```python
from build123d import *

# Parameters (mm, degrees)
SKETCH1_R           = 32.5
BOSS_EXTRUDE1_DEPTH = 2.25
SKETCH15_W          = 12.75
SKETCH15_H          = 3.5
CUT_EXTRUDE6_DEPTH  = 17
SKETCH17_W          = 21.5
SKETCH17_H          = 3.5
CUT_EXTRUDE7_DEPTH  = 12
SKETCH19_R          = 1
CUT_EXTRUDE9_DEPTH  = 16
FILLET4_R           = 0.5
FILLET5_R           = 0.5
SKETCH21_R          = 6.125
CUT_EXTRUDE11_DEPTH = 13
FILLET8_R           = 0.75


with BuildPart() as part:
    # Sketch1 → Boss-Extrude1 (new body)
    with BuildSketch(Plane(origin=(0, 0, 0), x_dir=(1, 0, 0), z_dir=(0, 1, 0))):
        Circle(SKETCH1_R)
    extrude(amount=BOSS_EXTRUDE1_DEPTH)

    # Sketch15 → Cut-Extrude6 (cut)
    with BuildSketch(Plane(origin=(0.067128405, 2.25, -0.501790944), x_dir=(1, 0, 0), z_dir=(0, 1, 0))):
        Polygon((-13.916501725, 15.395911949), (-20.291501725, 4.354088051), (-23.322590638, 6.104088051), (-16.947590638, 17.145911949), align=None)
        with Locations((0, 21.5)):
            Rectangle(SKETCH15_W, SKETCH15_H)
        Polygon((-20.291501725, -4.354088051), (-13.916501725, -15.395911949), (-16.947590638, -17.145911949), (-23.322590638, -6.104088051), align=None)
        with Locations((0, -21.5)):
            Rectangle(SKETCH15_W, SKETCH15_H)
        Polygon((13.916501725, -15.395911949), (20.291501725, -4.354088051), (23.322590638, -6.104088051), (16.947590638, -17.145911949), align=None)
        Polygon((20.291501725, 4.354088051), (13.916501725, 15.395911949), (16.947590638, 17.145911949), (23.322590638, 6.104088051), align=None)
    extrude(amount=-CUT_EXTRUDE6_DEPTH, mode=Mode.SUBTRACT)

    # Sketch17 → Cut-Extrude7 (cut)
    with BuildSketch(Plane(origin=(0.067128405, 2.25, -0.501790944), x_dir=(1, 0, 0), z_dir=(0, 1, 0))):
        Polygon((-17.715410458, -22.641027784), (-28.465410458, -4.021481603), (-25.434321545, -2.271481603), (-14.684321545, -20.891027784), align=None)
        with Locations((0, -24.912509387)):
            Rectangle(SKETCH17_W, SKETCH17_H)
        Polygon((-28.465410458, 4.021481603), (-17.715410458, 22.641027784), (-14.684321545, 20.891027784), (-25.434321545, 2.271481603), align=None)
        with Locations((0, 24.912509387)):
            Rectangle(SKETCH17_W, SKETCH17_H)
        Polygon((17.715410458, 22.641027784), (28.465410458, 4.021481603), (25.434321545, 2.271481603), (14.684321545, 20.891027784), align=None)
        Polygon((28.465410458, -4.021481603), (17.715410458, -22.641027784), (14.684321545, -20.891027784), (25.434321545, -2.271481603), align=None)
    extrude(amount=-CUT_EXTRUDE7_DEPTH, mode=Mode.SUBTRACT)

    # Sketch19 → Cut-Extrude9 (cut)
    with BuildSketch(Plane(origin=(0, 2.25, 0), x_dir=(1, 0, 0), z_dir=(0, 1, 0))):
        with Locations((-9.476258541, 17.306577458)):
            Circle(SKETCH19_R)
        with Locations((9.476258541, -17.306577458)):
            Circle(SKETCH19_R)
    extrude(amount=-CUT_EXTRUDE9_DEPTH, mode=Mode.SUBTRACT)

    # Fillet4
    fillet4_edges = [part.edges().sort_by_distance(p)[0] for p in [
        (-10.476258541, 2.25, -17.306577458),
        (8.476258541, 2.25, 17.306577458),
    ]]
    fillet(fillet4_edges, radius=FILLET4_R)

    # Fillet5
    fillet5_edges = [part.edges().sort_by_distance(p)[0] for p in [
        (-10.476258541, 0, -17.306577458),
        (8.476258541, 0, 17.306577458),
    ]]
    fillet(fillet5_edges, radius=FILLET5_R)

    # Sketch21 → Cut-Extrude11 (cut)
    with BuildSketch(Plane(origin=(0, 2.25, 0), x_dir=(1, 0, 0), z_dir=(0, 1, 0))):
        Circle(SKETCH21_R)
    extrude(amount=-CUT_EXTRUDE11_DEPTH, mode=Mode.SUBTRACT)

    # Fillet8
    fillet8_edges = [part.edges().sort_by_distance(p)[0] for p in [
        (-32.5, 2.25, 0),
    ]]
    fillet(fillet8_edges, radius=FILLET8_R)


solid = part.part
```
Design review of the part built by this model. Coordinates are the model's own, in mm. Give positions to 0.01 mm unless a question says otherwise; leave off trailing zeros. Order: outer loops, then holes, each group sorted by start corner. A loop starts at its lowest first (then second) coordinate and runs counter-clockwise, first axis right, second up. Notation, with made-up numbers: (64.25, 63.25) - (93.25, 63.25) arc R3 cw to (93.25, 67.25) - close; hole circle Ø6 at (87, 62.5). An arc over 180 degrees is marked (long way). Use a Markdown table: item, result. Add a question column.
(1) Add section C-C on x = 27. Give the number of separate pieces and of enclosed holes in the cut face, then the cut area to 3 significant figures.
(2) Wall thickness on probe 1 along Z at (x, y) = (-7, 1.5); probe 2 along Z at (x, y) = (-14.5, 1.25); probe 3 along X at (y, z) = (0.5, -22): over which ranges is each line inside the solid? List them lowest first. Write a range as [from, to].
(3) Add section B-B on z = 0. Give the boundary of the cut face in (x, y) (3 decimals).
(4) Mouldability with a two-part tool opening along X and no side actions: class faces 1 (the face through (21.857, 1.141, -5.721)), 2 (the face through (0, 2.25, 7)) as +X half, -X half, draft (parallel to the pull), parting line (faces both ways), or undercut.
(5) Add section A-A on x = 0. Give the boundary of the cut face in (y, z) (3 decimals), then the cut area to 3 significant figures.
(6) Clearance check with flat-ended pins moving along their axes: P1, Ø1.1, axis at y = 1, z = 24.5, coming from the -X side; P2, Ø1.1, axis at y = 1, z = -24.5, coming from the +X side; P3, Ø1.1, axis at y = 1, z = 24, coming from the +X side; P4, Ø4, axis at x = 13.5, z = -14, coming from the -Y side. State where each tip first meets the part, or that it passes through.
Report:
| question | item | result |
|---|---|---|
| 1 | separate pieces | 3 |
| 1 | enclosed holes | 0 |
| 1 | area | 65.0 mm² |
| 2 | probe 1 | z = [-31.74, -27.16], [-23.66, 22.66], [26.16, 31.74] |
| 2 | probe 2 | z = [-29.09, -16.27], [-14.77, 13.77], [15.27, 29.09] |
| 2 | probe 3 | x = [-23.92, -18.31], [-15.67, -6.31], [6.44, 15.8], [18.44, 23.92] |
| 3 | outline | (-32.5, 0) - (-6.125, 0) - (-6.125, 2.25) - (-31.75, 2.25) arc R0.75 ccw to (-32.5, 1.5) - close; (6.125, 0) - (32.5, 0) - (32.5, 1.5) arc R0.75 ccw to (31.75, 2.25) - (6.125, 2.25) - close |
| 4 | face 1 | undercut |
| 4 | face 2 | draft |
| 5 | outline | (0, -32.5) - (1.5, -32.5) arc R0.75 ccw to (2.25, -31.75) - (2.25, -27.164) - (0, -27.164) - close; (0, -20.252) - (2.25, -20.252) - (2.25, -6.125) - (0, -6.125) - close; (0, 6.125) - (2.25, 6.125) - (2.25, 19.248) - (0, 19.248) - close; (0, 26.161) - (2.25, 26.161) - (2.25, 31.75) arc R0.75 ccw to (1.5, 32.5) - (0, 32.5) - close |
| 5 | area | 87.3 mm² |
| 6 | P1 | stops at x = -21.97 |
| 6 | P2 | stops at x = 21.97 |
| 6 | P3 | stops at x = 22.5 |
| 6 | P4 | stops at y = 0 |
